from build123d import *

# Parameters (mm, degrees)
SKETCH_1_W          = 195
SKETCH_1_H          = 10
EXTRUDE_1_DEPTH     = 4
SKETCH_2_W          = 22
SKETCH_2_H          = 8
CUT_EXTRUDE_1_DEPTH = 3
SKETCH_3_W          = 5
SKETCH_3_H          = 5
CUT_EXTRUDE_2_DEPTH = 2


with BuildPart() as part:
    # 草图1 → 凸台-拉伸1 (new body)
    with BuildSketch(Plane(origin=(0, 0, 0), x_dir=(1, 0, 0), z_dir=(0, 1, 0))):
        Rectangle(SKETCH_1_W, SKETCH_1_H)
    extrude(amount=EXTRUDE_1_DEPTH)

    # 草图2 → 切除-拉伸1 (cut)
    with BuildSketch(Plane(origin=(0, 4, 0), x_dir=(1, 0, 0), z_dir=(0, 1, 0))):
        with Locations((-81.5, 0)):
            Rectangle(SKETCH_2_W, SKETCH_2_H)
    extrude(amount=-CUT_EXTRUDE_1_DEPTH, mode=Mode.SUBTRACT)

    # 草图3 → 切除-拉伸2 (cut)
    with BuildSketch(Plane(origin=(0, 4, 0), x_dir=(1, 0, 0), z_dir=(0, 1, 0))):
        with Locations((92.5, 0)):
            Rectangle(SKETCH_3_W, SKETCH_3_H)
        with Locations((47.14, 0)):
            Rectangle(SKETCH_3_W, SKETCH_3_H)
        with Locations((-13.22, 0)):
            Rectangle(SKETCH_3_W, SKETCH_3_H)
        with Locations((32.14, 0)):
            Rectangle(SKETCH_3_W, SKETCH_3_H)
    extrude(amount=-CUT_EXTRUDE_2_DEPTH, mode=Mode.SUBTRACT)


solid = part.part
Verification items for the finished model (mm, model axes). A direction names the side the tool comes from. Coordinates: 2 decimals unless noted, no trailing zeros. Order: outer loops, then holes, each group sorted by start corner. A loop starts at its lowest first (then second) coordinate and runs counter-clockwise, first axis right, second up.
Item 1: Access from +Z, -Z, +X, -X, +Y, -Y to the whole of each face (thin tool, end or side, straight path). Record for faces 1 (the face through (-82, 1, 0)), 2 (the face through (-1, 2, 5)).
Filled in:
face 1: +Y
face 2: +Z, +X, -X, +Y, -Y
Item 2: Section check B-B, the plane x = 47.5. Enter the section's corners in (y, z).
Filled in:
outline: (0, -5) - (4, -5) - (4, -2.5) - (2, -2.5) - (2, 2.5) - (4, 2.5) - (4, 5) - (0, 5) - close
Item 3: Material ranges on L1, parallel to X at y = 2.7, z = -1; L2, parallel to X at y = 1.2, z = 2; L3, parallel to Z at x = 45.5, y = 3.85, recorded low to high.
Filled in:
L1: x = -97.5 to -92.5, -70.5 to -15.72, -10.72 to 29.64, 34.64 to 44.64, 49.64 to 90, 95 to 97.5
L2: x = -97.5 to -92.5, -70.5 to 97.5
L3: z = -5 to -2.5, 2.5 to 5
Item 4: Release check for a two-part mould opening along X. For faces 3 (the face through (-97.5, 2, 0)), 4 (the face through (-1, 0, 0)), 5 (the face through (-70.5, 3, 0)) record: +X half, -X half, draft (parallel to the pull), parting line (faces both ways), or undercut.
Filled in:
face 3: -X half
face 4: draft
face 5: undercut
Item 5: Depth check by flat-ended pin: pin 1 (2.5 mm diameter, centred on x = 47.5, z = -1, fed in from +Y); pin 2 (2.5 mm diameter, centred on x = -83.5, z = 0.5, fed in from +Y); pin 3 (2 mm diameter, centred on x = 24.5, z = 1, fed in from -Y). Enter the tip coordinate at first touch or a pass-through.
Filled in:
pin 1: stops at y = 2
pin 2: stops at y = 1
pin 3: stops at y = 0
Item 6: Section check A-A, the plane y = 3.35. Enter the section's corners in (x, z), then the cut area to 3 significant figures.
Filled in:
outline: (-97.5, -5) - (97.5, -5) - (97.5, 5) - (-97.5, 5) - close; hole (-92.5, -4) - (-70.5, -4) - (-70.5, 4) - (-92.5, 4) - close; hole (-15.72, -2.5) - (-10.72, -2.5) - (-10.72, 2.5) - (-15.72, 2.5) - close; hole (29.64, -2.5) - (34.64, -2.5) - (34.64, 2.5) - (29.64, 2.5) - close; hole (44.64, -2.5) - (49.64, -2.5) - (49.64, 2.5) - (44.64, 2.5) - close; hole (90, -2.5) - (95, -2.5) - (95, 2.5) - (90, 2.5) - close
area: 1,670 mm2
